Geometry: final body of the model. Coordinates: model frame, mm. Coordinates: 2 decimals unless noted, no trailing zeros. Order: outer loops, then holes, each group sorted by start corner. A loop starts at its lowest first (then second) coordinate and runs counter-clockwise, first axis right, second up. Notation, with made-up numbers: (-20.5, 45) -> (-2.5, 45) arc R26 ccw to (-2.5, 79) -> close; hole circle Ø8 at (56, -32.75). An arc over 180 degrees is marked (long way). Use one line per item in the form item = value.
```python
from build123d import *

# Parameters (mm, degrees)
F1_R     = 75.730372
F2_DEPTH = 100
F3_R     = 10
F4_SIZE  = 15


with BuildPart() as f2:
    # F1 (on face) → F2 (new body)
    with BuildSketch(Plane.XZ):
        Circle(F1_R)
    extrude(amount=F2_DEPTH)

    # F3
    f3_edges = [f2.edges().sort_by_distance(p)[0] for p in [
        (-75.730372, 0, 0),
    ]]
    fillet(f3_edges, radius=F3_R)

    # F4
    f4_edges = [f2.edges().sort_by_distance(p)[0] for p in [
        (-75.730372, -100, 0),
    ]]
    chamfer(f4_edges, length=F4_SIZE)


solid = f2.part
```
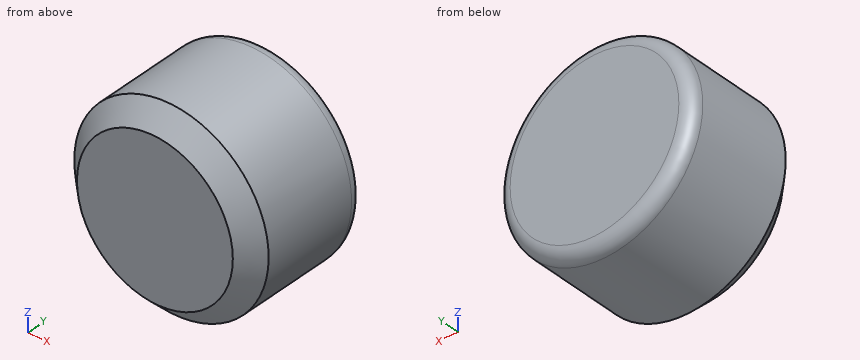
1) Contact query for flat-ended pins moving along their axis: P1, Ø6, axis at x = -6.5, y = -26, coming from the +Z side; P2, Ø10, axis at x = 12.5, y = -79.5, coming from the -Z side; P3, Ø8, axis at y = -10, z = 22.5, coming from the +X side. Output: stop coordinate, or through.
Results found:
P1 = 75.65
P2 = -75.36
P3 = 73.44
2) Material intervals for probe 1 along X at (y, z) = (-13, 1.5); probe 2 along Z at (x, y) = (60.5, -73); probe 3 along Z at (x, y) = (-34, -55), sorted ascending. Write a range as from..to.
Results found:
probe_1 = -75.72..75.72
probe_2 = -45.55..45.55
probe_3 = -67.67..67.67
3) Section B-B, the plane x = 0. Output: boundary loops of the cut face in (y, z).
Results found:
outline = (-100, -60.73) -> (-85, -75.73) -> (-10, -75.73) arc R10 ccw to (0, -65.73) -> (0, 65.73) arc R10 ccw to (-10, 75.73) -> (-85, 75.73) -> (-100, 60.73) -> close
4) Section C-C, the plane y = -55. Output: boundary loops of the cut face in (x, z).
Results found:
outline = circle Ø151.46 at (0, 0)
5) Section A-A, the plane z = 0. Output: boundary loops of the cut face in (x, y).
Results found:
outline = (-75.73, -85) -> (-60.73, -100) -> (60.73, -100) -> (75.73, -85) -> (75.73, -10) arc R10 ccw to (65.73, 0) -> (-65.73, 0) arc R10 ccw to (-75.73, -10) -> close
